```python
from build123d import *

# Parameters (mm, degrees)
F0_W         = 40
F0_H         = 70
F1_DEPTH     = 7
F2_R         = 5
F3_R         = 0.4991012629
F3_R_2       = 1.6336823689
F4_DEPTH     = 5
F5_T1_DEPTH  = 60
F5_T3_DEPTH  = 30
F5_T6_ANGLE  = 90
F5_T8_ANGLE  = 90
F5_T10_ANGLE = 90
F5_T12_ANGLE = 90
F5_T14_ANGLE = 90
F5_T16_ANGLE = 90
F5_T18_ANGLE = 90
F5_T20_ANGLE = 90
F6_R         = 3
F6_W         = 12
F6_H         = 1.5
F7_DEPTH     = 1


# Not quite as in the source:
# - a fillet or chamfer that OpenCascade refuses, or shapes differently, is made with other operations: its cross-section is extruded or revolved along the edge and cut away or added


with BuildPart() as f1:
    # F0 (on Top) → F1 (new body)
    with BuildSketch(Plane.XY):
        with Locations((20, 35)):
            Rectangle(F0_W, F0_H)
    extrude(amount=F1_DEPTH)

    # F2
    f2_edges = [f1.edges().sort_by_distance(p)[0] for p in [
        (40, 0, 3.5),
        (0, 0, 3.5),
        (40, 70, 3.5),
        (0, 70, 3.5),
    ]]
    fillet(f2_edges, radius=F2_R)

    # F3 (on face) → F4 (cut)
    with BuildSketch(Plane.XZ):
        with BuildLine():
            Line((21.5274822088, 4.6158107299), (17.7544243634, 4.6158107708))
            ThreePointArc((17.7544243634, 4.6158107708), (16.6386135926, 3.5), (17.7544243634, 2.3841892292))
            Line((17.7544243634, 2.3841892292), (21.5274822088, 2.3841892701))
            ThreePointArc((21.5274822088, 2.3841892701), (22.6432929266, 3.5), (21.5274822088, 4.6158107299))
        make_face()
        with Locations((26.0051637888, 3.5)):
            Circle(F3_R)
        with Locations((27.4651637888, 3.5)):
            Circle(F3_R)
        with Locations((28.9251637888, 3.5)):
            Circle(F3_R)
        with Locations((30.3851637888, 3.5)):
            Circle(F3_R)
        with Locations((31.8451637888, 3.5)):
            Circle(F3_R)
        with Locations((9.854494594, 3.5)):
            Circle(F3_R_2)
    extrude(amount=-F4_DEPTH, mode=Mode.SUBTRACT)

    # F5: fillet of radius 3 on 16 edges, made by hand

    # F5_s2 → F5_t1 (cut)
    with BuildSketch(Plane.XZ.offset(-65)):
        with BuildLine():
            ThreePointArc((0, 4), (0.8786796564, 6.1213203436), (3, 7))
            Line((3, 7), (0, 7))
            Line((0, 7), (0, 4))
        make_face()
        with BuildLine():
            ThreePointArc((0, 3), (0.8786796564, 0.8786796564), (3, 0))
            Line((3, 0), (0, 0))
            Line((0, 0), (0, 3))
        make_face()
        with BuildLine():
            ThreePointArc((37, 0), (39.1213203436, 0.8786796564), (40, 3))
            Line((40, 3), (40, 0))
            Line((40, 0), (37, 0))
        make_face()
        with BuildLine():
            ThreePointArc((37, 7), (39.1213203436, 6.1213203436), (40, 4))
            Line((40, 4), (40, 7))
            Line((40, 7), (37, 7))
        make_face()
    extrude(amount=F5_T1_DEPTH, mode=Mode.SUBTRACT)

    # F5_s4 → F5_t3 (cut)
    with BuildSketch(Plane.YZ.offset(5)):
        with BuildLine():
            ThreePointArc((67, 0), (69.1213203436, 0.8786796564), (70, 3))
            Line((70, 3), (70, 0))
            Line((70, 0), (67, 0))
        make_face()
        with BuildLine():
            ThreePointArc((3, 0), (0.8786796564, 0.8786796564), (0, 3))
            Line((0, 3), (0, 0))
            Line((0, 0), (3, 0))
        make_face()
        with BuildLine():
            ThreePointArc((67, 7), (69.1213203436, 6.1213203436), (70, 4))
            Line((70, 4), (70, 7))
            Line((70, 7), (67, 7))
        make_face()
        with BuildLine():
            ThreePointArc((3, 7), (0.8786796564, 6.1213203436), (0, 4))
            Line((0, 4), (0, 7))
            Line((0, 7), (3, 7))
        make_face()
    extrude(amount=F5_T3_DEPTH, mode=Mode.SUBTRACT)

    # F5_s5 → F5_t6 (revolve, cut)
    with BuildSketch(Plane.XZ.offset(-65)):
        with BuildLine():
            ThreePointArc((3, 0), (0.8786796564, 0.8786796564), (0, 3))
            Line((0, 3), (0, 0))
            Line((0, 0), (3, 0))
        make_face()
    revolve(axis=Axis((5, 65, 0), (0, 0, -1)), revolution_arc=F5_T6_ANGLE, mode=Mode.SUBTRACT)

    # F5_s7 → F5_t8 (revolve, cut)
    with BuildSketch(Plane.XZ.offset(-5)):
        with BuildLine():
            ThreePointArc((3, 0), (0.8786796564, 0.8786796564), (0, 3))
            Line((0, 3), (0, 0))
            Line((0, 0), (3, 0))
        make_face()
    revolve(axis=Axis((5, 5, 0), (0, 0, 1)), revolution_arc=F5_T8_ANGLE, mode=Mode.SUBTRACT)

    # F5_s9 → F5_t10 (revolve, cut)
    with BuildSketch(Plane.XZ.offset(-65)):
        with BuildLine():
            ThreePointArc((37, 0), (39.1213203436, 0.8786796564), (40, 3))
            Line((40, 3), (40, 0))
            Line((40, 0), (37, 0))
        make_face()
    revolve(axis=Axis((35, 65, 0), (0, 0, 1)), revolution_arc=F5_T10_ANGLE, mode=Mode.SUBTRACT)

    # F5_s11 → F5_t12 (revolve, cut)
    with BuildSketch(Plane.YZ.offset(35)):
        with BuildLine():
            ThreePointArc((3, 0), (0.8786796564, 0.8786796564), (0, 3))
            Line((0, 3), (0, 0))
            Line((0, 0), (3, 0))
        make_face()
    revolve(axis=Axis((35, 5, 0), (0, 0, 1)), revolution_arc=F5_T12_ANGLE, mode=Mode.SUBTRACT)

    # F5_s13 → F5_t14 (revolve, cut)
    with BuildSketch(Plane.XZ.offset(-65)):
        with BuildLine():
            ThreePointArc((0, 4), (0.8786796564, 6.1213203436), (3, 7))
            Line((3, 7), (0, 7))
            Line((0, 7), (0, 4))
        make_face()
    revolve(axis=Axis((5, 65, 7), (0, 0, -1)), revolution_arc=F5_T14_ANGLE, mode=Mode.SUBTRACT)

    # F5_s15 → F5_t16 (revolve, cut)
    with BuildSketch(Plane.XZ.offset(-5)):
        with BuildLine():
            ThreePointArc((0, 4), (0.8786796564, 6.1213203436), (3, 7))
            Line((3, 7), (0, 7))
            Line((0, 7), (0, 4))
        make_face()
    revolve(axis=Axis((5, 5, 7), (0, 0, 1)), revolution_arc=F5_T16_ANGLE, mode=Mode.SUBTRACT)

    # F5_s17 → F5_t18 (revolve, cut)
    with BuildSketch(Plane.XZ.offset(-65)):
        with BuildLine():
            ThreePointArc((37, 7), (39.1213203436, 6.1213203436), (40, 4))
            Line((40, 4), (40, 7))
            Line((40, 7), (37, 7))
        make_face()
    revolve(axis=Axis((35, 65, 7), (0, 0, 1)), revolution_arc=F5_T18_ANGLE, mode=Mode.SUBTRACT)

    # F5_s19 → F5_t20 (revolve, cut)
    with BuildSketch(Plane.YZ.offset(35)):
        with BuildLine():
            ThreePointArc((3, 7), (0.8786796564, 6.1213203436), (0, 4))
            Line((0, 4), (0, 7))
            Line((0, 7), (3, 7))
        make_face()
    revolve(axis=Axis((35, 5, 7), (0, 0, 1)), revolution_arc=F5_T20_ANGLE, mode=Mode.SUBTRACT)

    # F6 (on face) → F7 (cut)
    with BuildSketch(Plane.XY.offset(7)):
        with Locations((20, 10.0415023044)):
            Circle(F6_R)
        with Locations((20, 61.25)):
            Rectangle(F6_W, F6_H)
    extrude(amount=-F7_DEPTH, mode=Mode.SUBTRACT)


solid = f1.part
```
Input: part model. Units: mm. Frame: model coordinates. A direction names the side the tool comes from. Coordinates: 2 decimals unless noted, no trailing zeros. Write each loop counter-clockwise with the first axis right and the second up, starting at its lowest first coordinate (ties: lowest second). Pieces come first, ordered by that corner, then holes. Notation, with made-up numbers: M 47,21 L 68,21 A30 ccw 68,60 Z; hole C -35.75,6 d9. An arc over 180 degrees is marked long. Use one line per item in the form item = value.
Q1. Draft query along X for faces 4 (the face through (10.61, 2.46, 2.05)), 5 (the face through (39.1, 35.42, 0.86)), 6 (the face through (19.79, 69.1, 6.14)), 7 (the face through (20, 2, 2.384)). Return one class per face: released by +X, released by -X, zero draft, split by the parting line, or undercut.
Answer below:
face_4 = undercut
face_5 = released by +X
face_6 = zero draft
face_7 = undercut
Q2. Section C-C (x = 6). Return loops of the section in (y, z), plus the area to 3 significant figures.
Answer below:
outline = M 0,3 A3 ccw 3,0 L 67,0 A3 ccw 70,3 L 70,4 A3 ccw 67,7 L 3,7 A3 ccw 0,4 Z
area = 482 mm²
Q3. Section B-B (y = 24). Return loops of the section in (x, z), plus the area to 3 significant figures.
Answer below:
outline = M 0,3 A3 ccw 3,0 L 37,0 A3 ccw 40,3 L 40,4 A3 ccw 37,7 L 3,7 A3 ccw 0,4 Z
area = 272 mm²
Q4. First-contact query: pin 1 (0.8 mm diameter, centred on x = 27.5, z = 3.5, fed in from -Y); pin 2 (2 mm diameter, centred on x = 29, z = 6, fed in from +Y); pin 3 (0.5 mm diameter, centred on x = 19.5, z = 6.5, fed in from +Y). Flat tips, straight axial feed; report the tip coordinate or a pass-through.
Answer below:
pin_1 = 5
pin_2 = 69.83
pin_3 = 68.98
Q5. Set-up query: faces 1 (the face through (20, 35, 7)), 2 (the face through (20, 10, 6)), 3 (the face through (20, 5, 4)). Return all of +Z, -Z, +X, -X, +Y, -Y with unobstructed straight access to the full face (end or side cutting, diameter ignored); none if empty.
Answer below:
face_1 = +Z, +X, -X, +Y, -Y
face_2 = +Z
face_3 = -Y
Q6. Section A-A (x = 20). Return loops of the section in (y, z), plus the area to 3 significant figures.
Answer below:
outline = M 0.06,2.38 A3 ccw 3,0 L 67,0 A3 ccw 70,3 L 70,4 A3 ccw 67,7 L 62,7 L 62,6 L 60.5,6 L 60.5,7 L 13.04,7 L 13.04,6 L 7.04,6 L 7.04,7 L 3,7 A3 ccw 0.06,4.62 L 5,4.62 L 5,2.38 Z
area = 464 mm²
Q7. Material intervals for probe 1 along Y at (x, z) = (20, 6.6); probe 2 along X at (y, z) = (64, 4.25); probe 3 along Y at (x, z) = (17, 3), sorted ascending. Write a range as from..to.
Answer below:
probe_1 = 1.5..7.04, 13.04..60.5, 62..68.5
probe_2 = 0.01..39.99
probe_3 = 5..70
Q8. Section D-D (y = 8.5). Return loops of the section in (x, z).
Answer below:
outline = M 0,3 A3 ccw 3,0 L 37,0 A3 ccw 40,3 L 40,4 A3 ccw 37,7 L 22.57,7 L 22.57,6 L 17.43,6 L 17.43,7 L 3,7 A3 ccw 0,4 Z
